from build123d import *

# Parameters (mm, degrees)
SKETCH1_R           = 5.7759727
SKETCH1_R_2         = 12.7
BOSS_EXTRUDE1_DEPTH = 2.5


with BuildPart() as part:
    # Sketch1 → Boss-Extrude1 (new body)
    with BuildSketch(Plane.YZ):
        with BuildLine():
            Line((-25.399999937, -12.125972668), (-25.399999937, 12.125972668))
            ThreePointArc((-25.399999937, 12.125972668), (0, 37.525972605), (25.399999936, 12.125972668))
            Line((25.399999936, 12.125972668), (25.399999937, -12.125972668))
            ThreePointArc((25.399999937, -12.125972668), (0, -37.525972605), (-25.399999937, -12.125972668))
        make_face()
        with Locations(Location((0, 19.049999968, 0), (0, 0, 270))):
            Circle(SKETCH1_R, mode=Mode.SUBTRACT)
        with Locations(Location((0, -12.125972668, 0), (0, 0, 270))):
            Circle(SKETCH1_R_2, mode=Mode.SUBTRACT)
    extrude(amount=BOSS_EXTRUDE1_DEPTH)


solid = part.part
Build history of the part. All positions in model axes, mm. Coordinates: 2 decimals unless noted, no trailing zeros. Order: outer loops, then holes, each group sorted by start corner. A loop starts at its lowest first (then second) coordinate and runs counter-clockwise, first axis right, second up. Notation, with made-up numbers: (45, 60.25) - (96, 60.25) arc R27 cw to (96, 93.25) - close; hole circle Ø11 at (-20, -26). An arc over 180 degrees is marked (long way). Write item = value, one per line. Start each with the question number.
1) Wall check: line 1 along Z through (x, y) = (1.1, 4.5); line 2 along Y through (x, z) = (1.1, 19.05); line 3 along Y through (x, z) = (2.25, 15.5). Give the ranges that are in metal, low to high. Write a range as from..to.
2) Saw through at D-D on y = 10.5. Write the cut outline in (x, z).
3) Two-plate mould, pull along Z, no slides. Class faces 1 (the face through (1.23, -7.73, -2.05)), 2 (the face through (1, 25.4, 0)), 3 (the face through (1.23, -0.56, 37.52)), 4 (the face through (1.23, 0.56, -37.52)): pulls with the +Z half, pulls with the -Z half, needs draft (parallel to the pull), parting line crosses it, or undercut.
4) Flat gauge pin, fed straight in: pin 1 Ø1 at (x, z) = (2, -29) entering from -Y. Where does the tip first touch, or does it go through?
5) Saw through at C-C on x = 1.4. Write the cut outline in (y, z), then the cut area to 3 significant figures.
6) Saw through at B-B on z = -2.5. Write the cut outline in (x, y).
7) Saw through at A-A on y = 0. Write the cut outline in (x, z).
From the geometry:
q1.line_1 = -37.12..-24, -0.25..15.43, 22.67..37.12
q1.line_2 = -24.44..-5.78, 5.78..24.44
q1.line_3 = -25.17..-4.56, 4.56..25.17
q2.outline = (0, -35.25) - (2.5, -35.25) - (2.5, -19.27) - (0, -19.27) - close; (0, -4.98) - (2.5, -4.98) - (2.5, 35.25) - (0, 35.25) - close
q3.face_1 = undercut
q3.face_2 = needs draft
q3.face_3 = pulls with the +Z half
q3.face_4 = pulls with the -Z half
q4.pin_1 = -19.42
q5.outline = (-25.4, -12.13) arc R25.4 ccw to (25.4, -12.13) - (25.4, 12.13) arc R25.4 ccw to (-25.4, 12.13) - close; hole circle Ø25.4 at (0, -12.13); hole circle Ø11.55 at (0, 19.05)
q5.area = 2,650 mm^2
q6.outline = (0, -25.4) - (2.5, -25.4) - (2.5, -8.28) - (0, -8.28) - close; (0, 8.28) - (2.5, 8.28) - (2.5, 25.4) - (0, 25.4) - close
q7.outline = (0, -37.53) - (2.5, -37.53) - (2.5, -24.83) - (0, -24.83) - close; (0, 0.57) - (2.5, 0.57) - (2.5, 13.27) - (0, 13.27) - close; (0, 24.83) - (2.5, 24.83) - (2.5, 37.53) - (0, 37.53) - close
